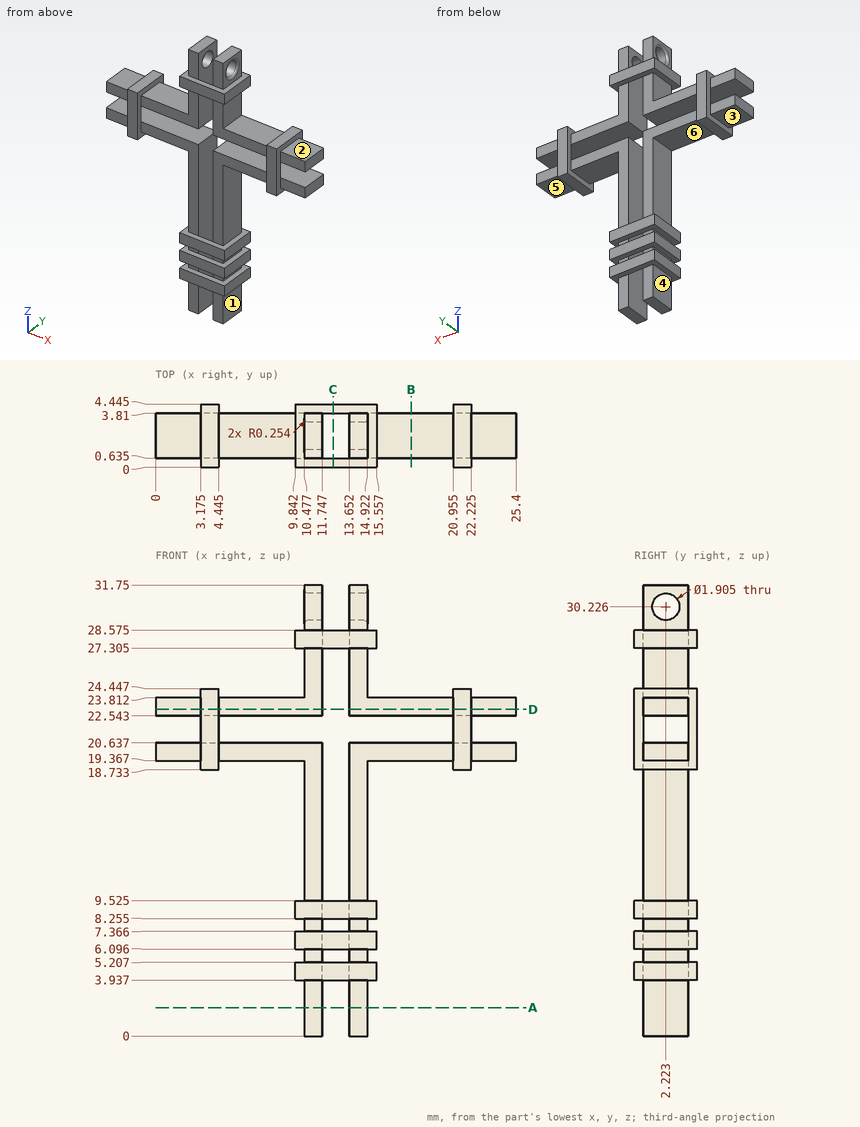
Can you work these out from the drawing? Everything is in mm from the part's minimum corner. A direction names the side the tool comes from. Give positions to 0.01 mm unless a question says otherwise; leave off trailing zeros. Order: outer loops, then holes, each group sorted by start corner. A loop starts at its lowest first (then second) coordinate and runs counter-clockwise, first axis right, second up.
1. Will these pins go through, and if not, where does the flat tip stop? P1, Ø1, axis at y = 2.5, z = 8.5, coming from the -X side; P2, Ø0.6, axis at x = 24.5, z = 23, coming from the +Y side; P3, Ø2.5, axis at x = 18, y = 2, coming from the +Z side.
2. Suppose I cut it at C-C (x = 12.5). Give the number of separate pieces and of enclosed holes in the cut face.
3. Suppose I cut it at A-A (z = 2). List the corners of the cut face in (x, y) for me (1 decimal).
4. Suppose I cut it at B-B (x = 18). List the corners of the cut face in (y, z) for me (1 decimal).
5. Suppose I cut it at D-D (z = 23). List the corners of the cut face in (x, y) for me (1 decimal).
6. We'd pull the mould along X, two halves only. Please class the marked faces 4, 5 and 6: pulls with the +X half, pulls with the -X half, needs draft (parallel to the pull), parting line crosses it, or undercut.
7. For the marked faces 1, 2 and 3, which set-ups out of +Z, -Z, +X, -X, +Y, -Y let a thin tool reach every point of the face, with its end or its side?
8. I need wall thicknesses on L1, parallel to X at y = 1.9, z = 19 (1 decimal); L2, parallel to Z at x = 11.25, y = 3.85 (1 decimal); L3, parallel to X at y = 3.1, z = 26.5. Which ranges of each line are inside material? Lowest first, please.
Solved:
1. P1: stops at x = 9.84
1. P2: stops at y = 3.81
1. P3: stops at z = 23.81
2. separate pieces: 8
2. enclosed holes: 0
3. outline: (10.5, 0.6) - (11.7, 0.6) - (11.7, 3.8) - (10.5, 3.8) - close; (13.7, 0.6) - (14.9, 0.6) - (14.9, 3.8) - (13.7, 3.8) - close
4. outline: (0.6, 19.4) - (3.8, 19.4) - (3.8, 20.6) - (0.6, 20.6) - close; (0.6, 22.5) - (3.8, 22.5) - (3.8, 23.8) - (0.6, 23.8) - close
5. outline: (0, 0.6) - (3.2, 0.6) - (3.2, 0) - (4.4, 0) - (4.4, 0.6) - (11.7, 0.6) - (11.7, 3.8) - (4.4, 3.8) - (4.4, 4.4) - (3.2, 4.4) - (3.2, 3.8) - (0, 3.8) - close; (13.7, 0.6) - (21, 0.6) - (21, 0) - (22.2, 0) - (22.2, 0.6) - (25.4, 0.6) - (25.4, 3.8) - (22.2, 3.8) - (22.2, 4.4) - (21, 4.4) - (21, 3.8) - (13.7, 3.8) - close
6. face 4: pulls with the -X half
6. face 5: needs draft
6. face 6: undercut
7. face 1: -Z, +X, +Y, -Y
7. face 2: +Z, +X, +Y, -Y
7. face 3: -Z, -X, +Y, -Y
8. L1: x = 3.2 to 4.4, 10.5 to 11.7, 13.7 to 14.9, 21 to 22.2
8. L2: z = 3.9 to 5.2, 6.1 to 7.4, 8.3 to 9.5, 27.3 to 28.6
8. L3: x = 10.48 to 11.75, 13.65 to 14.92
